The listing builds one solid part. Answer for the finished solid, in the listing's coordinates (mm). A direction names the side the tool comes from. Give positions to 0.01 mm unless a question says otherwise; leave off trailing zeros. Write each loop counter-clockwise with the first axis right and the second up, starting at its lowest first coordinate (ties: lowest second). Pieces come first, ordered by that corner, then holes. Notation, with made-up numbers: (-27.75, 45.5) - (-3.75, 45.5) arc R21 ccw to (-3.75, 71.5) - close; hole circle Ø11 at (-2, -4). An arc over 180 degrees is marked (long way). Answer as CSV lines item,"result". Start each with the question number.
(1) Find section C-C (x = 27). Write down the section's boundary in (y, z), then the cut area to 3 significant figures.
(2) For a pull along X with two mould halves and no side action, classify faces 4 (the face through (34, -13, 19)), 5 (the face through (23, -48, 1)), 6 (the face through (16, -42, 1)), 7 (the face through (46, -46, 3)) as pulls with the +X half, pulls with the -X half, needs draft (parallel to the pull), parting line crosses it, or undercut.
(3) Straight lines are drawn through the part: probe 1 along Y at (x, z) = (27, 0.95); probe 2 along Z at (x, y) = (44.5, -19.5); probe 3 along Y at (x, z) = (33, 10.75). For each, find the intervals that lie inside material, in ascending order.
(4) For faces 1 (the face through (35, -36.2, 3)), 2 (the face through (30, -34, 1)), 3 (the face through (40, -24, 19)), determine the directions among +Z, -Z, +X, -X, +Y, -Y from which every point of the face is accessible in a straight line to the end or side of a thin tool.
(5) Find section D-D (z = 15.5). Write down the section's boundary in (x, y).
(6) Find section A-A (x = 7). Write down the section's boundary in (y, z), then the cut area to 3 significant figures.
(7) Each of these flat-tipped pins is pushed along its axis until it touches: pin 1 Ø1.6 at (x, z) = (35, 2.5) entering from +Y; pin 2 Ø12 at (y, z) = (-40, 15.5) entering from -X; pin 3 Ø1.2 at (x, y) = (27, -24) entering from +Z; pin 4 Ø5 at (y, z) = (-27.5, 9.5) entering from -X. Where does it stop, or does it pass through?
(8) Find section B-B (y = -45). Write down the section's boundary in (x, z).
from build123d import *

# Parameters (mm, degrees)
SKETCH1_W           = 58
SKETCH1_H           = 48
BOSS_EXTRUDE1_DEPTH = 2
SKETCH2_R           = 1
SKETCH2_W           = 27
SKETCH2_H           = 16
CUT_EXTRUDE1_DEPTH  = 2
SKETCH3_W           = 54
SKETCH3_H           = 2
BOSS_EXTRUDE2_DEPTH = 18
CUT_EXTRUDE2_DEPTH  = 2
BOSS_EXTRUDE3_DEPTH = 46
BOSS_EXTRUDE4_DEPTH = 2
CUT_EXTRUDE3_DEPTH  = 13
SKETCH8_W           = 2
SKETCH8_H           = 48
BOSS_EXTRUDE5_DEPTH = 12


with BuildPart() as part:
    # Sketch1 → Boss-Extrude1 (new body)
    with BuildSketch(Plane.XY):
        with Locations((29, -24)):
            Rectangle(SKETCH1_W, SKETCH1_H)
    extrude(amount=BOSS_EXTRUDE1_DEPTH)

    # Sketch2 → Cut-Extrude1 (cut)
    with BuildSketch(Plane.XY.offset(2)):
        with Locations((5, -45)):
            Circle(SKETCH2_R)
        with Locations((27, -45)):
            Circle(SKETCH2_R)
        with Locations((5, -24)):
            Circle(SKETCH2_R)
        with Locations((27, -24)):
            Circle(SKETCH2_R)
        with Locations((16.5, -34)):
            Rectangle(SKETCH2_W, SKETCH2_H)
    extrude(amount=-CUT_EXTRUDE1_DEPTH, mode=Mode.SUBTRACT)

    # Sketch3 → Boss-Extrude2 (add)
    with BuildSketch(Plane.XY.offset(2)):
        with Locations((31, -1)):
            Rectangle(SKETCH3_W, SKETCH3_H)
    extrude(amount=BOSS_EXTRUDE2_DEPTH)

    # Sketch4 → Cut-Extrude2 (cut)
    with BuildSketch(Plane(origin=(0, 0, 0), x_dir=(1, 0, 0), z_dir=(0, 1, 0))):
        Polygon((4, -2), (34, -20), (4, -20), align=None)
    extrude(amount=-CUT_EXTRUDE2_DEPTH, mode=Mode.SUBTRACT)

    # Sketch5 → Boss-Extrude3 (add)
    with BuildSketch(Plane.XZ.offset(2)):
        Polygon((58, 20), (34, 20), (34, 18), (56, 18), (56, 2), (58, 2), (58, 18), align=None)
    extrude(amount=BOSS_EXTRUDE3_DEPTH)

    # Sketch6 → Boss-Extrude4 (add)
    with BuildSketch(Plane.XY.offset(2)):
        with BuildLine():
            Line((36, -36.2), (34, -36.2))
            ThreePointArc((34, -36.2), (37.527046669, -44.614867795), (46, -48))
            Line((46, -48), (57, -48))
            Line((57, -48), (57, -36.2))
            Line((57, -36.2), (56, -36.2))
            ThreePointArc((56, -36.2), (46, -46), (36, -36.2))
        make_face()
    extrude(amount=BOSS_EXTRUDE4_DEPTH)

    # Sketch7 → Cut-Extrude3 (cut)
    with BuildSketch(Plane.XY.offset(20)):
        with BuildLine():
            Line((58, -48), (58, -36.2))
            ThreePointArc((58, -36.2), (54.497222311, -27.64371576), (46, -24))
            Line((46, -24), (34, -24))
            Line((34, -24), (34, -48))
            Line((34, -48), (58, -48))
        make_face()
    extrude(amount=-CUT_EXTRUDE3_DEPTH, mode=Mode.SUBTRACT)

    # Sketch8 → Boss-Extrude5 (add)
    with BuildSketch(Plane.ZY):
        with Locations((1, -24)):
            Rectangle(SKETCH8_W, SKETCH8_H)
    extrude(amount=BOSS_EXTRUDE5_DEPTH)


solid = part.part
Result set:
1,outline,"(-48, 0) - (-46, 0) - (-46, 2) - (-48, 2) - close; (-44, 0) - (-42, 0) - (-42, 2) - (-44, 2) - close; (-26, 0) - (-25, 0) - (-25, 2) - (-26, 2) - close; (-23, 0) - (0, 0) - (0, 15.8) - (-2, 15.8) - (-2, 2) - (-23, 2) - close"
1,area,"83.6 mm^2"
2,face 4,"pulls with the -X half"
2,face 5,"needs draft"
2,face 6,"undercut"
2,face 7,"undercut"
3,probe 1,"-48 to -46, -44 to -42, -26 to -25, -23 to 0"
3,probe 2,"0 to 2, 18 to 20"
3,probe 3,"-2 to 0"
4,face 1,"+Z, -X"
4,face 2,"+Z, -Z"
4,face 3,"+Z, -X, -Y"
5,outline,"(26.5, -2) - (56, -2) - (56, -29.51) arc R12.2 cw to (58, -36.2) - (58, 0) - (26.5, 0) - close"
6,outline,"(-48, 0) - (-42, 0) - (-42, 2) - (-48, 2) - close; (-26, 0) - (0, 0) - (0, 3.8) - (-2, 3.8) - (-2, 2) - (-26, 2) - close"
6,area,"67.6 mm^2"
7,pin 1,"y = 0"
7,pin 2,"x = 57.8"
7,pin 3,"through"
7,pin 4,"x = 56"
8,outline,"(-12, 0) - (4, 0) - (4, 2) - (-12, 2) - close; (6, 0) - (26, 0) - (26, 2) - (6, 2) - close; (28, 0) - (58, 0) - (58, 7) - (56, 7) - (56, 4) - (50.36, 4) - (50.36, 2) - (41.64, 2) - (41.64, 4) - (37.94, 4) - (37.94, 2) - (28, 2) - close"
